from build123d import *

# Parameters (mm, degrees)
SKETCH1_W          = 115
SKETCH1_H          = 115
BASE_DEPTH         = 5
SKETCH2_W          = 115
SKETCH2_H          = 15
SKETCH2_W_2        = 105
SKETCH2_H_2        = 5.16
FRAME1_DEPTH       = 5
FRAME2_START       = -5
FRAME2_DEPTH       = 5
FRAME3_START       = -110
SKETCH2_4_W        = 115
SKETCH2_4_H        = 15
SKETCH2_4_W_2      = 105
SKETCH2_4_H_2      = 5.16
FRAME3_DEPTH       = 5
FRAME4_START       = -110
FRAME4_DEPTH       = 5
ANGLED_TRACK_DEPTH = 1.67


with BuildPart() as part:
    # Sketch1 → Base (new body)
    with BuildSketch(Plane(origin=(0, 0, 0), x_dir=(1, 0, 0), z_dir=(0, 1, 0))):
        Rectangle(SKETCH1_W, SKETCH1_H)
    extrude(amount=BASE_DEPTH)

    # Sketch2 → Frame1 (add)
    with BuildSketch(Plane.ZY.offset(57.5)):
        with Locations((0, 12.5)):
            Rectangle(SKETCH2_W, SKETCH2_H)
        with Locations((0, 12.5)):
            Rectangle(SKETCH2_W_2, SKETCH2_H_2, mode=Mode.SUBTRACT)
    extrude(amount=-FRAME1_DEPTH)

    # Sketch4 → Frame2 (add)
    with BuildSketch(Plane(origin=(0, 0, -57.5), x_dir=(-1, 0, 0), z_dir=(0, 0, -1)).offset(FRAME2_START)):
        Polygon((-57.5, 5), (-52.5, 5), (-52.5, 10.08), (52.5, 10.08), (52.5, 5), (57.5, 5), (57.5, 20), (52.5, 20), (52.5, 14.92), (-52.5, 14.92), (-52.5, 20), (-57.5, 20), align=None)
    extrude(amount=FRAME2_DEPTH)

    # Sketch2<4> → Frame3 (add)
    with BuildSketch(Plane.ZY.offset(57.5).offset(FRAME3_START)):
        with Locations((0, 12.5)):
            Rectangle(SKETCH2_4_W, SKETCH2_4_H)
        with Locations((0, 12.5)):
            Rectangle(SKETCH2_4_W_2, SKETCH2_4_H_2, mode=Mode.SUBTRACT)
    extrude(amount=-FRAME3_DEPTH)

    # Sketch4<3> → Frame4 (add)
    with BuildSketch(Plane(origin=(0, 0, -57.5), x_dir=(-1, 0, 0), z_dir=(0, 0, -1)).offset(FRAME4_START)):
        Polygon((-57.5, 5), (-52.5, 5), (-52.5, 10.08), (52.5, 10.08), (52.5, 5), (57.5, 5), (57.5, 20), (52.5, 20), (52.5, 14.92), (-52.5, 14.92), (-52.5, 20), (-57.5, 20), align=None)
    extrude(amount=-FRAME4_DEPTH)

    # Sketch7 → Angled Track (cut)
    with BuildSketch(Plane(origin=(0, 5, 0), x_dir=(1, 0, 0), z_dir=(0, 1, 0))):
        Polygon((52.5, -51.264920156), (-51.264920156, 52.5), (-52.5, 52.5), (-52.5, 51.264920156), (51.264920156, -52.5), (52.5, -52.5), align=None)
    extrude(amount=-ANGLED_TRACK_DEPTH, mode=Mode.SUBTRACT)


solid = part.part
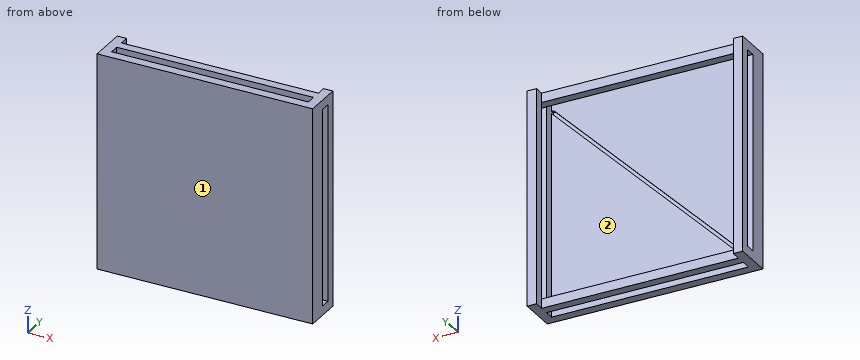
Geometry: final body of the model. Coordinates: model frame, mm. Face numbers are marked on the shaded views. Give positions to 0.01 mm unless a question says otherwise; leave off trailing zeros. Order: outer loops, then holes, each group sorted by start corner. A loop starts at its lowest first (then second) coordinate and runs counter-clockwise, first axis right, second up. Notation, with made-up numbers: (2.25, 15.5) -> (24.25, 15.5) arc R23 ccw to (24.25, 33.5) -> close; hole circle Ø6 at (21, 88.5). An arc over 180 degrees is marked (long way). Put each result on its own line as item: value.
Q1. Material intervals for L1, parallel to X at y = 7, z = 24; L2, parallel to Y at x = -31.5, z = 32, sorted ascending.
Here are the results:
L1: x = -57.5 to -52.5, 52.5 to 57.5
L2: y = 0 to 5
Q2. Section B-B, the plane x = 48.5. Return loops of the section in (y, z).
Here are the results:
outline: (0, -57.5) -> (5, -57.5) -> (5, 47.26) -> (3.33, 47.26) -> (3.33, 49.74) -> (5, 49.74) -> (5, 57.5) -> (0, 57.5) -> close; (10.08, -57.5) -> (14.92, -57.5) -> (14.92, -52.5) -> (10.08, -52.5) -> close; (10.08, 52.5) -> (14.92, 52.5) -> (14.92, 57.5) -> (10.08, 57.5) -> close
Q3. Section C-C, the plane z = -8.5. Return loops of the section in (x, y), then the cut area to 3 significant figures.
Here are the results:
outline: (-57.5, 0) -> (57.5, 0) -> (57.5, 9.92) -> (52.5, 9.92) -> (52.5, 5) -> (-7.26, 5) -> (-7.26, 3.33) -> (-9.74, 3.33) -> (-9.74, 5) -> (-52.5, 5) -> (-52.5, 9.92) -> (-57.5, 9.92) -> close; (-57.5, 15.08) -> (-52.5, 15.08) -> (-52.5, 20) -> (-57.5, 20) -> close; (52.5, 15.08) -> (57.5, 15.08) -> (57.5, 20) -> (52.5, 20) -> close
area: 669 mm^2
Q4. Draft query along X for the marked faces 1 and 2. Return one class per face: released by +X, released by -X, zero draft, split by the parting line, or undercut.
Here are the results:
face 1: zero draft
face 2: undercut
Q5. Section A-A, the plane y = 8.25. Return loops of the section in (x, z).
Here are the results:
outline: (-57.5, -57.5) -> (-52.5, -57.5) -> (-52.5, 57.5) -> (-57.5, 57.5) -> close; (52.5, -57.5) -> (57.5, -57.5) -> (57.5, 57.5) -> (52.5, 57.5) -> close
Q6. Pin query (flat end, axial travel): pin 1 (4 mm diameter, centred on x = -1.5, z = 55.5, fed in from +Y); pin 2 (2.5 mm diameter, centred on x = 12.5, z = 56, fed in from -Y); pin 3 (6 mm diameter, centred on x = -45.5, z = -10.5, fed in from +Y). Return the tip coordinate at first contact, or that it passes through.
Here are the results:
pin 1: stops at y = 14.92
pin 2: stops at y = 0
pin 3: stops at y = 5
